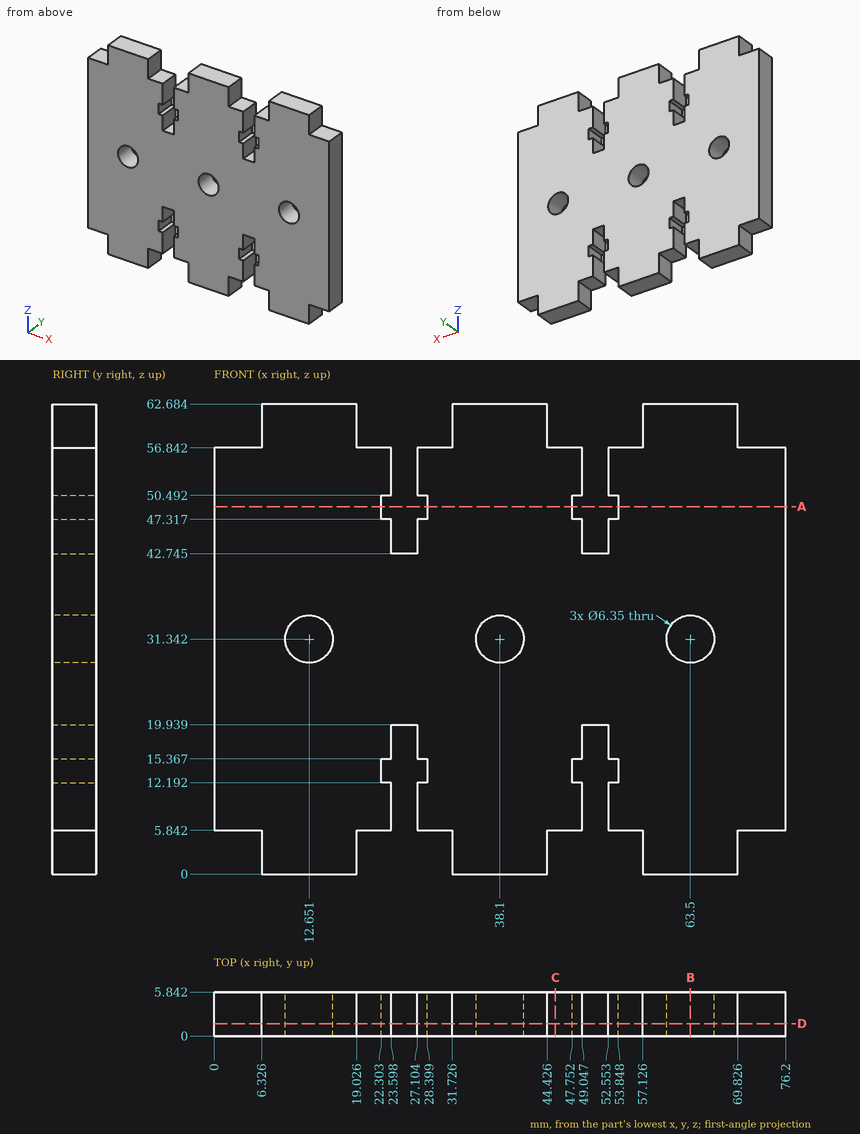
Can you work these out from the drawing? Everything is in mm from the part's minimum corner. Round coordinates to 2 decimals unless told otherwise and drop trailing zeros. Loops run counter-clockwise (first coordinate to the right, second up) from the corner with the lowest first, then second, coordinate; pieces in that order, holes last. Notation, with made-up numbers: (59.25, 87.25) -> (65.25, 87.25) arc R3 ccw to (65.25, 91.25) -> close; hole circle Ø11 at (85.25, 17.5). An arc over 180 degrees is marked (long way). Answer in a Markdown table with one row per item.
Item 1: Suppose I cut it at A-A, the plane z = 49. List the corners of the cut face in (x, y) for me.
Answer block:
| item | result |
|---|---|
| outline | (0, 0) -> (22.3, 0) -> (22.3, 5.84) -> (0, 5.84) -> close; (28.4, 0) -> (47.75, 0) -> (47.75, 5.84) -> (28.4, 5.84) -> close; (53.85, 0) -> (76.2, 0) -> (76.2, 5.84) -> (53.85, 5.84) -> close |
Item 2: Suppose I cut it at C-C, the plane x = 45.5. List the corners of the cut face in (y, z) for me.
Answer block:
| item | result |
|---|---|
| outline | (0, 5.84) -> (5.84, 5.84) -> (5.84, 56.84) -> (0, 56.84) -> close |
Item 3: Suppose I cut it at B-B, the plane x = 63.5. List the corners of the cut face in (y, z) for me.
Answer block:
| item | result |
|---|---|
| outline | (0, 0) -> (5.84, 0) -> (5.84, 28.17) -> (0, 28.17) -> close; (0, 34.52) -> (5.84, 34.52) -> (5.84, 62.68) -> (0, 62.68) -> close |
Item 4: Suppose I cut it at D-D, the plane y = 1.65. Give the number of separate pieces and of enclosed holes in the cut face, plus the area to 3 significant figures.
Answer block:
| item | result |
|---|---|
| separate pieces | 1 |
| enclosed holes | 3 |
| area | 4,010 mm² |
Item 5: Will these pins go through, and if not, where does the flat tip stop? P1, Ø1.4, axis at x = 27.5, y = 2, coming from the -Z side; P2, Ø1, axis at x = 48.5, y = 2.5, coming from the +Z side.
Answer block:
| item | result |
|---|---|
| P1 | z = 5.84 |
| P2 | z = 56.84 |
Item 6: If I drill on probe 1 along X at (y, z) = (2.6, 13.5); probe 2 along X at (y, z) = (2.75, 53); probe 3 along X at (y, z) = (4.95, 29.5) (1 decimal), over which ranges is the centre line in solid material (lowest first)?
Answer block:
| item | result |
|---|---|
| probe 1 | 0 to 22.3, 28.4 to 47.75, 53.85 to 76.2 |
| probe 2 | 0 to 23.6, 27.1 to 49.05, 52.55 to 76.2 |
| probe 3 | 0 to 10.1, 15.2 to 35.5, 40.7 to 60.9, 66.1 to 76.2 |
